Geometry check sheet. Reference: the model listing, model coordinates, mm. Face numbers are marked on the shaded views. A direction names the side the tool comes from. Give positions to 0.01 mm unless a question says otherwise; leave off trailing zeros. Write each loop counter-clockwise with the first axis right and the second up, starting at its lowest first coordinate (ties: lowest second). Pieces come first, ordered by that corner, then holes. Notation, with made-up numbers: (86, 65) - (113, 65) arc R28 cw to (113, 94) - close; hole circle Ø8 at (-26.5, -29). An arc over 180 degrees is marked (long way). Use a Markdown table: item, result.
```python
from build123d import *

# Parameters (mm, degrees)
SKETCH1_W           = 59
SKETCH1_H           = 94
SKETCH1_W_2         = 55
SKETCH1_H_2         = 90
EXTRUDE_THIN1_DEPTH = 26
SKETCH2_W           = 59
SKETCH2_H           = 94
BOSS_EXTRUDE1_DEPTH = 2


with BuildPart() as part:
    # Sketch1 → Extrude-Thin1 (new body)
    with BuildSketch(Plane.XY):
        with Locations((80.9055, -64.39)):
            Rectangle(SKETCH1_W, SKETCH1_H)
        with Locations((80.9055, -64.39)):
            Rectangle(SKETCH1_W_2, SKETCH1_H_2, mode=Mode.SUBTRACT)
    extrude(amount=EXTRUDE_THIN1_DEPTH)

    # Sketch2 → Boss-Extrude1 (add)
    with BuildSketch(Plane.XY.offset(26)):
        with Locations((80.9055, -64.39)):
            Rectangle(SKETCH2_W, SKETCH2_H)
    extrude(amount=BOSS_EXTRUDE1_DEPTH)


solid = part.part
```
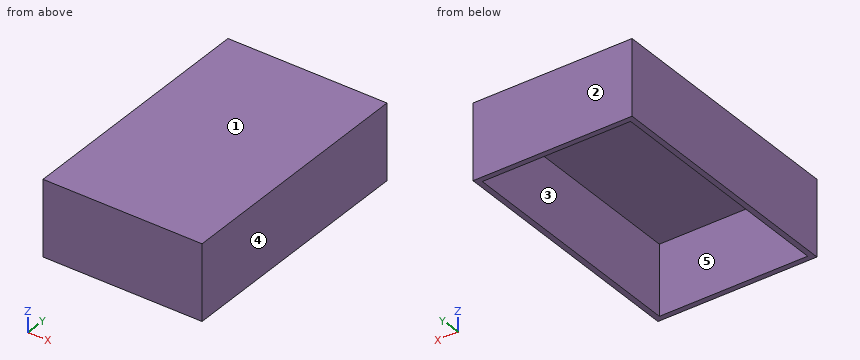
1) Section check C-C on y = -41. Record the boundary of the cut face in (x, z), then the cut area to 3 significant figures.
Working result:
| item | result |
|---|---|
| outline | (51.41, 0) - (53.41, 0) - (53.41, 26) - (108.41, 26) - (108.41, 0) - (110.41, 0) - (110.41, 28) - (51.41, 28) - close |
| area | 222 mm² |
2) Mould release check, pull along Y, two halves, no side actions. Record for the marked faces 1, 2 and 3: pulls with the +Y half, pulls with the -Y half, needs draft (parallel to the pull), parting line crosses it, or undercut.
Working result:
| item | result |
|---|---|
| face 1 | needs draft |
| face 2 | pulls with the +Y half |
| face 3 | undercut |
3) Section check A-A on z = 17.25. Record the boundary of the cut face in (x, y).
Working result:
| item | result |
|---|---|
| outline | (51.41, -111.39) - (110.41, -111.39) - (110.41, -17.39) - (51.41, -17.39) - close; hole (53.41, -109.39) - (108.41, -109.39) - (108.41, -19.39) - (53.41, -19.39) - close |
4) Material ranges on L1, parallel to X at y = -89, z = 10.5; L2, parallel to Y at x = 63, z = 24.25; L3, parallel to Z at x = 89, y = -69.5, recorded low to high. Write a range as from..to.
Working result:
| item | result |
|---|---|
| L1 | x = 51.41..53.41, 108.41..110.41 |
| L2 | y = -111.39..-109.39, -19.39..-17.39 |
| L3 | z = 26..28 |
5) Section check B-B on x = 106. Record the boundary of the cut face in (y, z).
Working result:
| item | result |
|---|---|
| outline | (-111.39, 0) - (-109.39, 0) - (-109.39, 26) - (-19.39, 26) - (-19.39, 0) - (-17.39, 0) - (-17.39, 28) - (-111.39, 28) - close |
6) Set-up check for the marked faces 4 and 5: record each of +Z, -Z, +X, -X, +Y, -Y from which the full face is reachable in a straight line by a thin tool's end or side.
Working result:
| item | result |
|---|---|
| face 4 | +Z, -Z, +X, +Y, -Y |
| face 5 | -Z |
